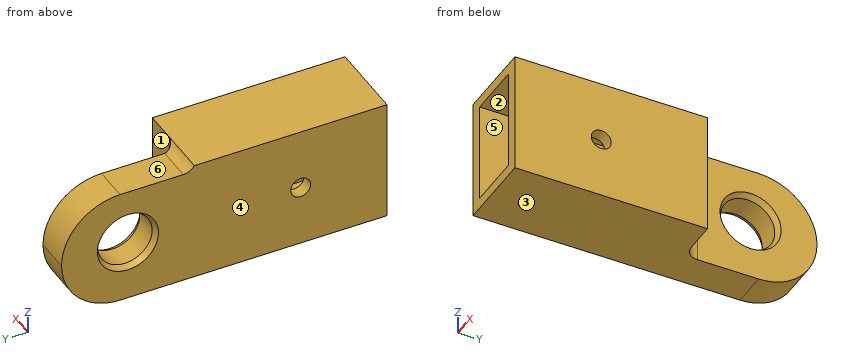
```python
from build123d import *
from OCP.BRepFilletAPI import BRepFilletAPI_MakeChamfer

# Parameters (mm, degrees)
SKETCH1_W           = 12
SKETCH1_H           = 18.5
BOSS_EXTRUDE1_DEPTH = 29
SKETCH2_W           = 8.2
SKETCH2_H           = 15.2
CUT_EXTRUDE1_DEPTH  = 23
SKETCH4_W           = 5.3
SKETCH4_H           = 17.6
BOSS_EXTRUDE2_DEPTH = 20
CUT_EXTRUDE2_REACH  = 52.314
SKETCH5_R           = 4.1
FILLET1_R           = 8.8
SKETCH6_R           = 1.5
CUT_EXTRUDE3_DEPTH  = 52.289009544
CHAMFER1_SIZE       = 0.5
CHAMFER1_SIZE2      = 0.866025404
FILLET6_R           = 2


# Some blends are built 0.0001 mm under size
with BuildPart() as part:
    # Sketch1 → Boss-Extrude1 (new body)
    with BuildSketch(Plane(origin=(0, 0, 0), x_dir=(1, 0, 0), z_dir=(0, 1, 0))):
        Rectangle(SKETCH1_W, SKETCH1_H)
    extrude(amount=BOSS_EXTRUDE1_DEPTH)

    # Sketch2 → Cut-Extrude1 (cut)
    with BuildSketch(Plane.XZ):
        Rectangle(SKETCH2_W, SKETCH2_H)
    extrude(amount=-CUT_EXTRUDE1_DEPTH, mode=Mode.SUBTRACT)

    # Sketch4 → Boss-Extrude2 (add)
    with BuildSketch(Plane(origin=(0, 29, 0), x_dir=(1, 0, 0), z_dir=(0, 1, 0))):
        with Locations((-3.35, 0.45)):
            Rectangle(SKETCH4_W, SKETCH4_H)
    extrude(amount=BOSS_EXTRUDE2_DEPTH)

    # Sketch5 → Cut-Extrude2 (cut, up to next)
    with BuildSketch(Plane(origin=(-0.7, 0, 0), x_dir=(0, 0, -1), z_dir=(1, 0, 0)), mode=Mode.PRIVATE) as cut_extrude2_sk1:
        with Locations((0, 39)):
            Circle(SKETCH5_R)
    cut_extrude2_tool1 = extrude(cut_extrude2_sk1.sketch, amount=-CUT_EXTRUDE2_REACH, mode=Mode.PRIVATE) & part.part
    add(cut_extrude2_tool1.solids().sort_by_distance((-0.7, 39, 0))[0], mode=Mode.SUBTRACT)

    # Fillet1
    fillet1_edges = [part.edges().sort_by_distance(p)[0] for p in [
        (-3.35, 49, -9.25),
        (-3.35, 49, 8.35),
    ]]
    fillet(fillet1_edges, radius=FILLET1_R - 0.0001)  # a hair under: the kernel refuses the full size

    # Sketch6 → Cut-Extrude3 (cut, through all)
    with BuildSketch(Plane(origin=(6, 0, 0), x_dir=(0, 0, -1), z_dir=(1, 0, 0))):
        with Locations((0, 13)):
            Circle(SKETCH6_R)
    extrude(amount=-CUT_EXTRUDE3_DEPTH, mode=Mode.SUBTRACT)

    # Chamfer1: one chamfer whose edges measure the first distance from different faces: ONE call of the kernel's chamfer builder (chamfer() names one face for all edges)
    chamfer1_edges_1 = [part.edges().sort_by_distance(p)[0] for p in [
        (-0.7, 39, 4.1),
    ]]
    chamfer1_side_1 = [part.faces().sort_by_distance(p)[0] for p in [
        (-0.7, 34.60005, 8.083586787),
    ]]
    chamfer1_edges_2 = [part.edges().sort_by_distance(p)[0] for p in [
        (-6, 39, 4.1),
    ]]
    chamfer1_side_2 = [part.faces().sort_by_distance(p)[0] for p in [
        (-6, 22.369672876, -0.180344797),
    ]]
    chamfer1 = BRepFilletAPI_MakeChamfer(part.part.solid().wrapped)
    for e in chamfer1_edges_1:
        chamfer1.Add(CHAMFER1_SIZE, CHAMFER1_SIZE2, e.wrapped, chamfer1_side_1[0].wrapped)  # the first distance lies on this face
    for e in chamfer1_edges_2:
        chamfer1.Add(CHAMFER1_SIZE, CHAMFER1_SIZE2, e.wrapped, chamfer1_side_2[0].wrapped)  # the first distance lies on this face
    add(Compound.cast(chamfer1.Shape()), mode=Mode.REPLACE)

    # Fillet6
    # the kernel refuses this fillet: 2 mm, written as the material it adds along each edge
    with BuildSketch(Plane(origin=(-0.7, 29, 8.35), x_dir=(1, 0, 0), z_dir=(0, 0, -1))) as fillet6_piece_1:
        with BuildLine():
            CenterArc((FILLET6_R, -FILLET6_R), FILLET6_R, 90, 90)
            Line((0, -FILLET6_R), (-FILLET6_R * 0.02, -FILLET6_R))
            Line((-FILLET6_R * 0.02, -FILLET6_R), (-FILLET6_R * 0.02, FILLET6_R * 0.02))
            Line((-FILLET6_R * 0.02, FILLET6_R * 0.02), (FILLET6_R, FILLET6_R * 0.02))
            Line((FILLET6_R, FILLET6_R * 0.02), (FILLET6_R, 0))
        make_face()
    extrude(amount=17.6)
    with BuildSketch(Plane(origin=(-6, 29, 8.35), x_dir=(0, 1.5316143415257847e-12, 1.0), z_dir=(1, 0, 0))) as fillet6_piece_2:
        with BuildLine():
            CenterArc((2, -1.670329309), FILLET6_R, 123.367012969, 56.632987031)
            Line((0, -1.670329309), (-0.04, -1.670329309))
            Line((-0.04, -1.670329309), (-0.04, 0))
            Line((-0.04, 0), (0, 0.04))
            ThreePointArc((0, 0.04), (0.45, 0.04), (0.878, 0.033406586))
            Line((0.878, 0.033406586), (0.9, 0))
        make_face()
    extrude(amount=5.3)
    with BuildSketch(Plane(origin=(-6, 29, 8.35), x_dir=(0, 1.5316143415257847e-12, 1.0), z_dir=(1, 0, 0))) as fillet6_piece_3a_section:
        with BuildLine():
            CenterArc((2, -1.670329309), FILLET6_R, 123.367012969, 56.632987031)
            Line((0, -1.670329309), (-0.04, -1.670329309))
            Line((-0.04, -1.670329309), (-0.04, 0))
            Line((-0.04, 0), (0, 0.04))
            ThreePointArc((0, 0.04), (0.45, 0.04), (0.878, 0.033406586))
            Line((0.878, 0.033406586), (0.9, 0))
        make_face()
    fillet6_piece_3a = extrude(amount=9.475823272, mode=Mode.PRIVATE)
    fillet6_piece_3a = split(fillet6_piece_3a, bisect_by=Plane(origin=(-0.7, 29.423174299, 8.582221018), z_dir=(1, 0, 0)), keep=Keep.TOP, mode=Mode.PRIVATE)
    with BuildSketch(Plane(origin=(-0.7, 29, 13.35), x_dir=(1, 0, 0), z_dir=(0, 0, -1))) as fillet6_piece_3b_section:
        with BuildLine():
            CenterArc((FILLET6_R, -FILLET6_R), FILLET6_R, 90, 90)
            Line((0, -FILLET6_R), (-FILLET6_R * 0.02, -FILLET6_R))
            Line((-FILLET6_R * 0.02, -FILLET6_R), (-FILLET6_R * 0.02, FILLET6_R * 0.02))
            Line((-FILLET6_R * 0.02, FILLET6_R * 0.02), (FILLET6_R, FILLET6_R * 0.02))
            Line((FILLET6_R, FILLET6_R * 0.02), (FILLET6_R, 0))
        make_face()
    fillet6_piece_3b = extrude(amount=22.6, mode=Mode.PRIVATE)
    fillet6_piece_3b = split(fillet6_piece_3b, bisect_by=Plane(origin=(-0.247209771, 29.452790229, 9.25), z_dir=(0, 0, -1)), keep=Keep.TOP, mode=Mode.PRIVATE)
    fillet6_piece_3b = split(fillet6_piece_3b, bisect_by=Plane(origin=(-0.247209771, 29.452790229, 8.35), z_dir=(0, 0, 1)), keep=Keep.TOP, mode=Mode.PRIVATE)
    fillet6_piece_3 = fillet6_piece_3a & fillet6_piece_3b
    add(fillet6_piece_3)


solid = part.part
```
Geometry: final body of the model. Coordinates: model frame, mm. Face numbers are marked on the shaded views. A direction names the side the tool comes from. Round coordinates to 2 decimals unless told otherwise and drop trailing zeros. Order: outer loops, then holes, each group sorted by start corner. A loop starts at its lowest first (then second) coordinate and runs counter-clockwise, first axis right, second up. Notation, with made-up numbers: (2, 77.5) - (37, 77.5) arc R23 cw to (37, 86.5) - close; hole circle Ø3 at (77, 29). An arc over 180 degrees is marked (long way). Write item = value, one per line. Start each with the question number.
Q1. Access query for the marked faces 1, 2 and 3. Directions: +Z, -Z, +X, -X, +Y, -Y. A direction counts if a zero-diameter tool reaches every point of the face in a straight line with its end or side. Return the directions, or none.
Q2. Ray query, line 1 (Y direction, x = 4.7, z = 0); line 2 (Z direction, x = -1, y = 20); line 3 (X direction, y = 11, z = 4). Return the intervals inside material, ascending. Write a range as from..to.
Q3. Pull-direction query (Z, two-part tool) for the marked faces 4, 5 and 6; classes: +Z half, -Z half, draft (parallel to the pull), parting line (faces both ways), or undercut.
Q4. Cut plane A-A on y = 39. Return the cut outline in (x, z).
Q5. Cut plane C-C on x = 3. Return the cut outline in (y, z), and give its area (3 significant figures).
Q6. Pin query (flat end, axial travel): pin 1 (6 mm diameter, centred on x = 2.5, z = 3.5, fed in from +Y); pin 2 (3 mm diameter, centred on y = 42.5, z = 2, fed in from -X); pin 3 (1.6 mm diameter, centred on x = -2, y = 33.5, fed in from +Z); pin 4 (4 mm diameter, centred on x = -1.5, z = 2.5, fed in from -Y). Return the tip coordinate at first contact, or that it passes through.
Q7. Cut plane D-D on z = 0. Return the cut outline in (x, y), and give its area (3 significant figures).
Q8. Cut plane B-B on y = 21.5. Return the cut outline in (x, z).
Outcome:
q1.face_1 = +Z, -Z, +X, +Y
q1.face_2 = -Y
q1.face_3 = -Z, +X, -X, +Y, -Y
q2.line_1 = 0..11.5, 14.5..29
q2.line_2 = -9.25..-7.6, 7.6..9.25
q2.line_3 = -6..-4.1, 4.1..6
q3.face_4 = draft
q3.face_5 = undercut
q3.face_6 = +Z half
q4.outline = (-6, -9.25) - (-0.7, -9.25) - (-0.7, -4.6) - (-1.57, -4.1) - (-5.13, -4.1) - (-6, -4.6) - close; (-6, 4.6) - (-5.13, 4.1) - (-1.57, 4.1) - (-0.7, 4.6) - (-0.7, 8.35) - (-6, 8.35) - close
q5.outline = (0, -9.25) - (29, -9.25) - (29, 9.25) - (0, 9.25) - (0, 7.6) - (23, 7.6) - (23, -7.6) - (0, -7.6) - close
q5.area = 187 mm^2
q6.pin_1 = 30.13
q6.pin_2 = -6
q6.pin_3 = 8.35
q6.pin_4 = 23
q7.outline = (-6, 0) - (-4.1, 0) - (-4.1, 11.5) - (-6, 11.5) - close; (-6, 14.5) - (-4.1, 14.5) - (-4.1, 23) - (4.1, 23) - (4.1, 14.5) - (6, 14.5) - (6, 29) - (1.3, 29) arc R2 cw to (-0.7, 31) - (-0.7, 34.4) - (-1.57, 34.9) - (-5.13, 34.9) - (-6, 34.4) - close; (-6, 43.6) - (-5.13, 43.1) - (-1.57, 43.1) - (-0.7, 43.6) - (-0.7, 48.99) - (-6, 48.99) - close; (4.1, 0) - (6, 0) - (6, 11.5) - (4.1, 11.5) - close
q7.area = 210 mm^2
q8.outline = (-6, -9.25) - (6, -9.25) - (6, 9.25) - (-6, 9.25) - close; hole (-4.1, -7.6) - (4.1, -7.6) - (4.1, 7.6) - (-4.1, 7.6) - close
